Study the drawing (mm; zero at the part's minimum x, y, z) and answer. A direction names the side the tool comes from. Coordinates: 2 decimals unless noted, no trailing zeros. Loops run counter-clockwise (first coordinate to the right, second up) from the corner with the lowest first, then second, coordinate; pieces in that order, holes last. Notation, with made-up numbers: (-18, 33.5) -> (-11, 33.5) arc R22 ccw to (-11, 46.5) -> close; hole circle Ø6 at (15, 65). An arc over 180 degrees is marked (long way). Answer as CSV lines item,"result".
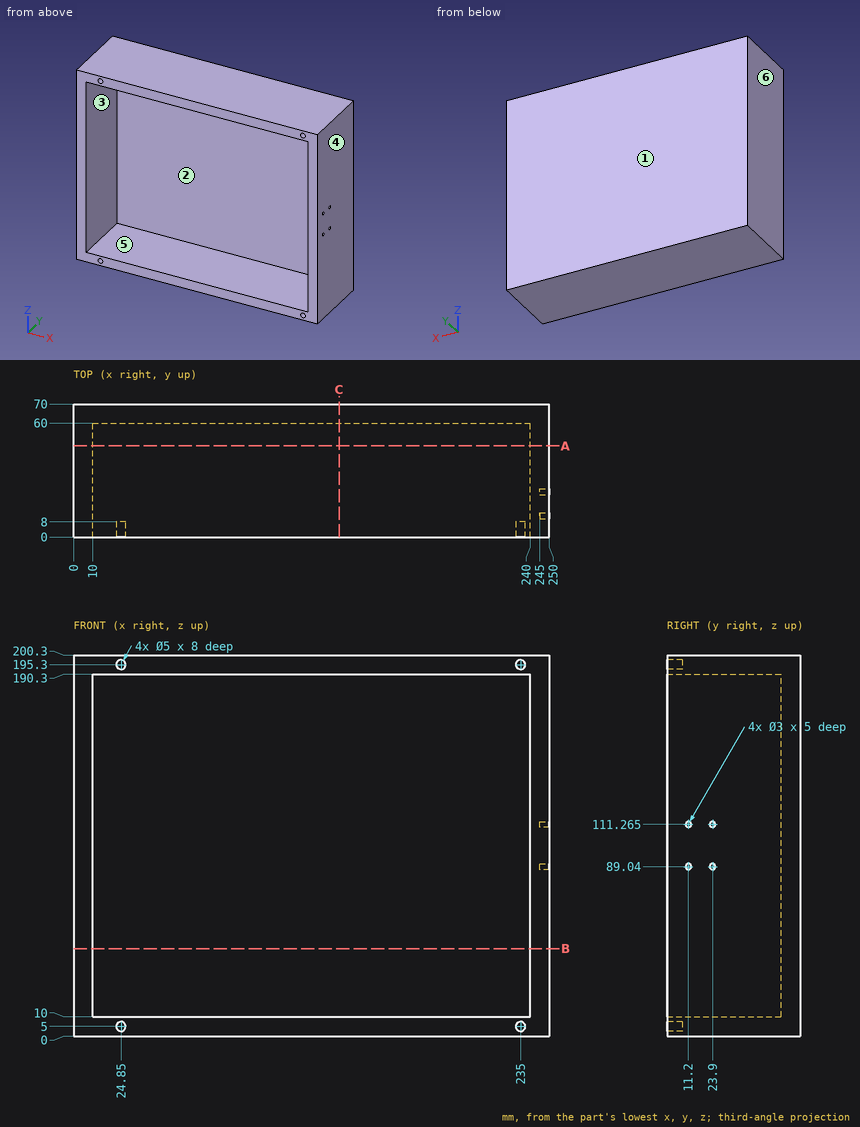
Q1. Find the intervals of material crossed by probe 1 along X at (y, z) = (2, 195); probe 2 along Z at (x, y) = (235, 4.75); probe 3 along Y at (x, z) = (248.4, 89.04), in increasing order. Write a range as [from, to].
Results:
probe 1,"x = [0, 22.37], [27.33, 232.52], [237.48, 250]"
probe 2,"z = [0, 2.5], [7.5, 10], [190.3, 192.8], [197.8, 200.3]"
probe 3,"y = [0, 9.7], [12.7, 22.4], [25.4, 70]"
Q2. For a pull along X with two mould halves and no side action, classify the marked faces 3, 4, 5 and 6 as pulls with the +X half, pulls with the -X half, needs draft (parallel to the pull), parting line crosses it, or undercut.
Results:
face 3,"undercut"
face 4,"pulls with the +X half"
face 5,"undercut"
face 6,"pulls with the -X half"
Q3. For the marked faces 1 and 2, determine the directions among +Z, -Z, +X, -X, +Y, -Y from which every point of the face is accessible in a straight line to the end or side of a thin tool.
Results:
face 1,"+Z, -Z, +X, -X, +Y"
face 2,"-Y"
Q4. Given pin 1 Ø2.5 at (y, z) = (23.9, 89.04) entering from +X; pin 2 Ø1.8 at (y, z) = (11.2, 89.04) entering from -X; pin 3 Ø1.5 at (x, z) = (222.5, 57) entering from -Y; pin 4 Ø4.5 at (x, z) = (24.85, 195.3) entering from -Y, each flat-ended and moving along its own axis, determine where each tip first touches the part or whether it passes through.
Results:
pin 1,"stops at x = 245"
pin 2,"stops at x = 0"
pin 3,"stops at y = 60"
pin 4,"stops at y = 8"
Q5. A cutting plane is placed at C-C, the plane x = 139.5. Write down the section's boundary in (y, z), and give its area (3 significant figures).
Results:
outline,"(0, 0) -> (70, 0) -> (70, 200.3) -> (0, 200.3) -> (0, 190.3) -> (60, 190.3) -> (60, 10) -> (0, 10) -> close"
area,"3,200 mm²"
Q6. A cutting plane is placed at B-B, the plane z = 46. Write down the section's boundary in (x, y), and give its area (3 significant figures).
Results:
outline,"(0, 0) -> (10, 0) -> (10, 60) -> (240, 60) -> (240, 0) -> (250, 0) -> (250, 70) -> (0, 70) -> close"
area,"3,700 mm²"
Q7. A cutting plane is placed at A-A, the plane y = 48. Write down the section's boundary in (x, z), and give its area (3 significant figures).
Results:
outline,"(0, 0) -> (250, 0) -> (250, 200.3) -> (0, 200.3) -> close; hole (10, 10) -> (240, 10) -> (240, 190.3) -> (10, 190.3) -> close"
area,"8,610 mm²"
